Input: part model. Units: mm. Frame: model coordinates. A direction names the side the tool comes from. Give positions to 0.01 mm unless a question says otherwise; leave off trailing zeros. Write each loop counter-clockwise with the first axis right and the second up, starting at its lowest first coordinate (ties: lowest second). Pieces come first, ordered by that corner, then holes. Notation, with made-up numbers: (-20.75, 5) - (-6.75, 5) arc R20 cw to (-6.75, 28) - close; hole circle Ø1 at (30.25, -1.75). An arc over 180 degrees is marked (long way). Answer as CSV lines item,"result".
Autodesk Inventor part; units mm, degrees
ref_plane "YZ Plane" through (0, 0, 0) normal (1, 0, 0) x (0, 1, 0)
ref_plane "XZ Plane" through (0, 0, 0) normal (0, 1, 0) x (-1, 0, 0)
ref_plane "XY Plane" through (0, 0, 0) normal (0, 0, 1) x (1, 0, 0)
sketch "Sketch1" plane through (0, 0, 0) normal (0, 0, 1) x (1, 0, 0)
  circle A0 centre (0, 0) radius 3.175
  dimension "d0" = 6.35
extrude "Extrusion1" add sketch "Sketch1" along normal blind 97.6
chamfer "Chamfer1" distance 0.3 angle 45 2 edges at (-3.175, 0, 97.6) (-3.175, 0, 0)
sketch "Sketch2" plane through (0, 0, 97.6) normal (0, 0, 1) x (1, 0, 0)
  circle A0 centre (0, 0) radius 0.5
  dimension "d6" = 1
extrude "Extrusion2" cut sketch "Sketch2" against normal blind 2
sketch "Sketch3" plane through (0, 0, 0) normal (0, 0, -1) x (-1, 0, 0)
  circle A0 centre (0, 0) radius 0.5
extrude "Extrusion3" cut sketch "Sketch3" against normal blind 2
sketch "Sketch4" plane through (0, 0, 97.6) normal (0, 0, 1) x (1, 0, 0)
  circle A0 centre (0, 0) radius 3.175
  line L0 (-1.7861, 2.625) -> (-1.675, 2.625)
  line L1 (-1.675, 2.625) -> (1.7861, 2.625)
  dimension "d11" = 2.625
extrude "Extrusion4" cut sketch "Sketch4" against normal blind 15 contours L1 L0 A0 picked at (0.4083, 2.7411)
properties part number "motorAxis" material "Stainless Steel"
Item 1: Ray query, line 1 (Y direction, x = 0, z = 1.1) (3 decimals); line 2 (Y direction, x = 0, z = 96.6) (3 decimals); line 3 (Y direction, x = -0.25, z = 66.5). Return the intervals inside material, ascending. Write a range as from..to.
The answers:
line 1,"-3.175..-0.5, 0.5..3.175"
line 2,"-3.175..-0.5, 0.5..2.625"
line 3,"-3.17..3.17"
Item 2: Contact query for flat-ended pins moving along their axis: pin 1 (0.8 mm diameter, centred on x = 0, y = 0, fed in from -Z); pin 2 (0.5 mm diameter, centred on x = 0, y = 0, fed in from +Z); pin 3 (1.1 mm diameter, centred on x = 1, z = 91, fed in from +Y) (3 decimals). Output: stop coordinate, or through.
The answers:
pin 1,"z = 2"
pin 2,"z = 95.6"
pin 3,"y = 2.625"
Item 3: Cut plane A-A on z = 50. Return the cut outline in (x, y) (3 decimals).
The answers:
outline,"circle Ø6.35 at (0, 0)"
Item 4: Reachability of faces 1 (the face through (-0.41, -3.15, 48.12)), 2 (the face through (0, 2.625, 90)) from +Z, -Z, +X, -X, +Y, -Y: full face, straight path, thin tool, end or side. Return the list, or none.
The answers:
face 1,"+Z, -Z"
face 2,"+Z, +X, -X, +Y"
